Work out the finished part from the listing and answer in its coordinate system (mm). A direction names the side the tool comes from. Give positions to 0.01 mm unless a question says otherwise; leave off trailing zeros. Loops run counter-clockwise (first coordinate to the right, second up) from the corner with the lowest first, then second, coordinate; pieces in that order, holes last. Notation, with made-up numbers: M 47.5,77.25 L 58.5,77.25 A36 cw 58.5,115.25 Z; hole C -38.5,81.5 d3. An arc over 180 degrees is marked long. Use a Markdown table: item, result.
```python
from build123d import *

# Parameters (mm, degrees)
F0_R     = 25
F0_R_2   = 3.517009594
F1_DEPTH = 5


with BuildPart() as f1:
    # F0 (on Right) → F1 (new body)
    with BuildSketch(Plane.YZ):
        Circle(F0_R)
        with BuildLine():
            add(Edge.make_bspline(
                [(-4.2770959996, -4.1764053417), (-4.7479386555, -4.2915002132), (-5.3150424766, -4.2915002132)],
                knots=[0, 0, 0, 1, 1, 1], degree=2))
            add(Edge.make_bspline(
                [(-5.3150424766, -4.2915002132), (-6.5183070416, -4.2915002132), (-7.2057373192, -3.5779120103)],
                knots=[0, 0, 0, 1, 1, 1], degree=2))
            add(Edge.make_bspline(
                [(-7.2057373192, -3.5779120103), (-7.8931675968, -2.8643238073), (-7.8931675968, -1.6024654896)],
                knots=[0, 0, 0, 1, 1, 1], degree=2))
            add(Edge.make_bspline(
                [(-7.8931675968, -1.6024654896), (-7.8931675968, -0.3740893162), (-7.4055838687, 0.7548867409)],
                knots=[0, 0, 0, 1, 1, 1], degree=2))
            add(Edge.make_bspline(
                [(-7.4055838687, 0.7548867409), (-6.9180001406, 1.883862798), (-6.1133823575, 2.5116530059)],
                knots=[0, 0, 0, 1, 1, 1], degree=2))
            add(Edge.make_bspline(
                [(-6.1133823575, 2.5116530059), (-5.3087645745, 3.1394432137), (-4.3419676544, 3.1394432137)],
                knots=[0, 0, 0, 1, 1, 1], degree=2))
            add(Edge.make_bspline(
                [(-4.3419676544, 3.1394432137), (-3.3416885899, 3.1394432137), (-2.8373637896, 2.7041753363)],
                knots=[0, 0, 0, 1, 1, 1], degree=2))
            add(Edge.make_bspline(
                [(-2.8373637896, 2.7041753363), (-2.3330389893, 2.2689074588), (-2.3330389893, 1.4904476011)],
                knots=[0, 0, 0, 1, 1, 1], degree=2))
            add(Edge.make_bspline(
                [(-2.3330389893, 1.4904476011), (-2.3330389893, 0.3143872784), (-3.4191160489, -0.356301927)],
                knots=[0, 0, 0, 1, 1, 1], degree=2))
            add(Edge.make_bspline(
                [(-3.4191160489, -0.356301927), (-4.5051931084, -1.0269911324), (-6.5266775777, -1.0269911324)],
                knots=[0, 0, 0, 1, 1, 1], degree=2))
            Line((-6.5266775777, -1.0269911324), (-6.7422188824, -1.0269911324))
            Line((-6.7422188824, -1.0269911324), (-6.7673304907, -1.5501496389))
            add(Edge.make_bspline(
                [(-6.7673304907, -1.5501496389), (-6.7673304907, -2.4060369556), (-6.3655447577, -2.8873427816)],
                knots=[0, 0, 0, 1, 1, 1], degree=2))
            add(Edge.make_bspline(
                [(-6.3655447577, -2.8873427816), (-5.9637590247, -3.3686486076), (-5.1204275121, -3.3686486076)],
                knots=[0, 0, 0, 1, 1, 1], degree=2))
            add(Edge.make_bspline(
                [(-5.1204275121, -3.3686486076), (-4.708178609, -3.3686486076), (-4.2729107315, -3.2504147852)],
                knots=[0, 0, 0, 1, 1, 1], degree=2))
            add(Edge.make_bspline(
                [(-4.2729107315, -3.2504147852), (-3.8376428541, -3.1321809627), (-3.19101894, -2.8182858588)],
                knots=[0, 0, 0, 1, 1, 1], degree=2))
            Line((-3.19101894, -2.8182858588), (-3.19101894, -3.7746196087))
            add(Edge.make_bspline(
                [(-3.19101894, -3.7746196087), (-3.8062533437, -4.0613104703), (-4.2770959996, -4.1764053417)],
                knots=[0, 0, 0, 1, 1, 1], degree=2))
        make_face(mode=Mode.SUBTRACT)
        with BuildLine():
            add(Edge.make_bspline(
                [(0.4574884846, 2.4781708614), (1.2746620718, 3.1394432137), (2.249829528, 3.1394432137)],
                knots=[0, 0, 0, 1, 1, 1], degree=2))
            add(Edge.make_bspline(
                [(2.249829528, 3.1394432137), (2.8504154935, 3.1394432137), (3.3212581494, 2.8150849397)],
                knots=[0, 0, 0, 1, 1, 1], degree=2))
            add(Edge.make_bspline(
                [(3.3212581494, 2.8150849397), (3.7921008053, 2.4907266656), (4.0536800586, 1.883862798)],
                knots=[0, 0, 0, 1, 1, 1], degree=2))
            Line((4.0536800586, 1.883862798), (4.1269222495, 1.883862798))
            Line((4.1269222495, 1.883862798), (4.5642827609, 3.0076072701))
            Line((4.5642827609, 3.0076072701), (5.3950584693, 3.0076072701))
            Line((5.3950584693, 3.0076072701), (3.8716208983, -4.1596642695))
            Line((3.8716208983, -4.1596642695), (3.0010851434, -4.1596642695))
            Line((3.0010851434, -4.1596642695), (3.1726811335, -2.7931742505))
            Line((3.1726811335, -2.7931742505), (3.1203652829, -2.7931742505))
            add(Edge.make_bspline(
                [(3.1203652829, -2.7931742505), (1.9484902282, -4.2915002132), (0.653149766, -4.2915002132)],
                knots=[0, 0, 0, 1, 1, 1], degree=2))
            add(Edge.make_bspline(
                [(0.653149766, -4.2915002132), (-0.2550534013, -4.2915002132), (-0.7719340058, -3.6438299821)],
                knots=[0, 0, 0, 1, 1, 1], degree=2))
            add(Edge.make_bspline(
                [(-0.7719340058, -3.6438299821), (-1.2888146102, -2.996159751), (-1.2888146102, -1.8703226449)],
                knots=[0, 0, 0, 1, 1, 1], degree=2))
            add(Edge.make_bspline(
                [(-1.2888146102, -1.8703226449), (-1.2888146102, -0.5101105279), (-0.8242498564, 0.6533939906)],
                knots=[0, 0, 0, 1, 1, 1], degree=2))
            add(Edge.make_bspline(
                [(-0.8242498564, 0.6533939906), (-0.3596851026, 1.8168985092), (0.4574884846, 2.4781708614)],
                knots=[0, 0, 0, 1, 1, 1], degree=2))
        make_face(mode=Mode.SUBTRACT)
        with BuildLine():
            Line((7.4751366913, 3.0076072701), (8.5863253592, 3.0076072701))
            Line((8.5863253592, 3.0076072701), (7.606972635, -1.5375938348))
            add(Edge.make_bspline(
                [(7.606972635, -1.5375938348), (7.4876924955, -2.119346094), (7.4876924955, -2.4457970021)],
                knots=[0, 0, 0, 1, 1, 1], degree=2))
            add(Edge.make_bspline(
                [(7.4876924955, -2.4457970021), (7.4876924955, -3.3812044118), (8.4503041475, -3.3812044118)],
                knots=[0, 0, 0, 1, 1, 1], degree=2))
            add(Edge.make_bspline(
                [(8.4503041475, -3.3812044118), (9.0257785047, -3.3812044118), (9.5813728387, -2.9888355319)],
                knots=[0, 0, 0, 1, 1, 1], degree=2))
            add(Edge.make_bspline(
                [(9.5813728387, -2.9888355319), (10.1369671726, -2.596466652), (10.5617718799, -1.8640447428)],
                knots=[0, 0, 0, 1, 1, 1], degree=2))
            add(Edge.make_bspline(
                [(10.5617718799, -1.8640447428), (10.9865765872, -1.1316228337), (11.210488428, -0.0978616248)],
                knots=[0, 0, 0, 1, 1, 1], degree=2))
            Line((11.210488428, -0.0978616248), (11.8633902442, 3.0076072701))
            Line((11.8633902442, 3.0076072701), (12.9494673038, 3.0076072701))
            Line((12.9494673038, 3.0076072701), (11.4385855369, -4.1596642695))
            Line((11.4385855369, -4.1596642695), (10.5303823695, -4.1596642695))
            Line((10.5303823695, -4.1596642695), (10.6726814833, -2.832934297))
            Line((10.6726814833, -2.832934297), (10.5952540243, -2.832934297))
            add(Edge.make_bspline(
                [(10.5952540243, -2.832934297), (9.9549080123, -3.6490615672), (9.372109436, -3.9702808902)],
                knots=[0, 0, 0, 1, 1, 1], degree=2))
            add(Edge.make_bspline(
                [(9.372109436, -3.9702808902), (8.7893108598, -4.2915002132), (8.167798554, -4.2915002132)],
                knots=[0, 0, 0, 1, 1, 1], degree=2))
            add(Edge.make_bspline(
                [(8.167798554, -4.2915002132), (7.3307449435, -4.2915002132), (6.8536243856, -3.8363523125)],
                knots=[0, 0, 0, 1, 1, 1], degree=2))
            add(Edge.make_bspline(
                [(6.8536243856, -3.8363523125), (6.3765038276, -3.3812044118), (6.3765038276, -2.5378728993)],
                knots=[0, 0, 0, 1, 1, 1], degree=2))
            add(Edge.make_bspline(
                [(6.3765038276, -2.5378728993), (6.3765038276, -2.1319018982), (6.5208955754, -1.4120357932)],
                knots=[0, 0, 0, 1, 1, 1], degree=2))
            Line((6.5208955754, -1.4120357932), (7.4751366913, 3.0076072701))
        make_face(mode=Mode.SUBTRACT)
        with BuildLine():
            Line((-13.9618062727, 5.401580596), (-11.509239194, 5.401580596))
            add(Edge.make_bspline(
                [(-11.509239194, 5.401580596), (-8.6841832587, 5.401580596), (-8.6841832587, 3.2043148685)],
                knots=[0, 0, 0, 1, 1, 1], degree=2))
            add(Edge.make_bspline(
                [(-8.6841832587, 3.2043148685), (-8.6841832587, 2.281463263), (-9.2523333968, 1.6473951531)],
                knots=[0, 0, 0, 1, 1, 1], degree=2))
            add(Edge.make_bspline(
                [(-9.2523333968, 1.6473951531), (-9.8204835349, 1.0133270431), (-10.8542447438, 0.8228973468)],
                knots=[0, 0, 0, 1, 1, 1], degree=2))
            Line((-10.8542447438, 0.8228973468), (-10.8542447438, 0.7580256919))
            add(Edge.make_bspline(
                [(-10.8542447438, 0.7580256919), (-10.1029891284, 0.5487622893), (-9.7001570784, 0.0350206359)],
                knots=[0, 0, 0, 1, 1, 1], degree=2))
            add(Edge.make_bspline(
                [(-9.7001570784, 0.0350206359), (-9.2973250284, -0.4787210175), (-9.2973250284, -1.1964944885)],
                knots=[0, 0, 0, 1, 1, 1], degree=2))
            add(Edge.make_bspline(
                [(-9.2973250284, -1.1964944885), (-9.2973250284, -2.5839108478), (-10.2913261908, -3.3717875587)],
                knots=[0, 0, 0, 1, 1, 1], degree=2))
            add(Edge.make_bspline(
                [(-10.2913261908, -3.3717875587), (-11.2853273532, -4.1596642695), (-12.9531566721, -4.1596642695)],
                knots=[0, 0, 0, 1, 1, 1], degree=2))
            Line((-12.9531566721, -4.1596642695), (-15.9811981079, -4.1596642695))
            Line((-15.9811981079, -4.1596642695), (-13.9618062727, 5.401580596))
        make_face(mode=Mode.SUBTRACT)
        with Locations((-4.4432776049, 19.0966390073)):
            Circle(F0_R_2, mode=Mode.SUBTRACT)
    extrude(amount=F1_DEPTH)


solid = f1.part
```
(1) A cutting plane is placed at A-A (y = 15). Write down the section's boundary in (x, z).
Entries:
| item | result |
|---|---|
| outline | M 0,-20 L 5,-20 L 5,20 L 0,20 Z |
(2) Which of the six approach directions +Z, -Z, +X, -X, +Y, -Y give full straight-line access (tool end or side, diameter ignored) to faces 4 (the flat face through (5, 5, 0)), 5 (the flat face through (2.465, 4.343, 2.438))?
Entries:
| item | result |
|---|---|
| face 4 | +Z, -Z, +X, +Y, -Y |
| face 5 | +X, -X |
(3) A cutting plane is placed at C-C (x = 4). Count the separate pieces of the cut face and the enclosed holes in it, and give its area (3 significant figures).
Entries:
| item | result |
|---|---|
| separate pieces | 1 |
| enclosed holes | 5 |
| area | 1,790 mm² |
(4) The mould has two halves that part along Y. Classify faces 1 (the flat face through (2.46, 11.53, 1.43)), 2 (the cylindrical face through (2.465, 23.846, 7.509)), 3 (the flat face through (0, 5, 0)): released by +Y, released by -Y, zero draft, split by the parting line, or undercut.
Entries:
| item | result |
|---|---|
| face 1 | undercut |
| face 2 | split by the parting line |
| face 3 | zero draft |
(5) A cutting plane is placed at B-B (z = -7). Write down the section's boundary in (x, y), and give its area (3 significant figures).
Entries:
| item | result |
|---|---|
| outline | M 0,-24 L 5,-24 L 5,24 L 0,24 Z |
| area | 240 mm² |
(6) Consider probe 1 along Y at (x, z) = (4.35, 20); probe 2 along Y at (x, z) = (4.55, 5); probe 3 along Z at (x, y) = (4.5, -12). Determine where each line is inside the solid, lowest interval first. Write a range as [from, to].
Entries:
| item | result |
|---|---|
| probe 1 | y = [-15, -7.84], [-1.04, 15] |
| probe 2 | y = [-24.49, -14.05], [-9.61, 24.49] |
| probe 3 | z = [-21.93, -4.09], [5.4, 21.93] |
(7) Given P1, Ø0.7, axis at x = 2, y = -12.5, coming from the -Z side; P2, Ø2.5, axis at x = 1.5, y = -14.5, coming from the +Z side; P3, Ø1.2, axis at x = 2.5, y = 12.5, coming from the -Z side, each flat-ended and moving along its own axis, determine where each tip first touches the part or whether it passes through.
Entries:
| item | result |
|---|---|
| P1 | stops at z = -21.85 |
| P2 | stops at z = 21.2 |
| P3 | stops at z = -21.99 |
